Can you work these out from the model? Positions are in its coordinate system, mm. Face numbers are marked on the shaded views. Give positions to 0.01 mm unless a question says otherwise; leave off trailing zeros. Order: outer loops, then holes, each group sorted by start corner. A loop starts at its lowest first (then second) coordinate and runs counter-clockwise, first axis right, second up. Notation, with made-up numbers: M 43.25,13 L 96.25,13 A24 cw 96.25,48 Z; hole C -16,60.25 d6. An arc over 180 degrees is marked long. Answer as a JSON object with one key per item and string values.
```python
from build123d import *

# Parameters (mm, degrees)
SKETCH1_R               = 10
BOSS_EXTRUDE1_DEPTH     = 30
SKETCH2_R               = 2.5
BOSS_EXTRUDE3_DEPTH     = 2
SHELL1_T                = -0.8
SKETCH3_R               = 0.5
CUT_EXTRUDE2_DEPTH      = 34.166247904
CUT_EXTRUDE2_DEPTH_BACK = 34.166247904


with BuildPart() as part:
    # Sketch1 → Boss-Extrude1 (new body)
    with BuildSketch(Plane.XY):
        Circle(SKETCH1_R)
    extrude(amount=BOSS_EXTRUDE1_DEPTH)

    # Sketch2 → Boss-Extrude3 (add)
    with BuildSketch(Plane.XY):
        Circle(SKETCH2_R)
    extrude(amount=-BOSS_EXTRUDE3_DEPTH)

    # Shell1
    shell1_openings = [part.faces().sort_by_distance(p)[0] for p in [
        (0, 0, 30),
        (0, 0, -2),
    ]]
    offset(amount=SHELL1_T, openings=shell1_openings, kind=Kind.INTERSECTION)

    # Sketch3 → Cut-Extrude2 (cut, two sides)
    with BuildSketch(Plane.XY) as cut_extrude2_sk:
        with Locations((5, 0)):
            Circle(SKETCH3_R)
        with Locations((0, -5)):
            Circle(SKETCH3_R)
        with Locations((-5, 0)):
            Circle(SKETCH3_R)
        with Locations((0, 5)):
            Circle(SKETCH3_R)
    extrude(amount=CUT_EXTRUDE2_DEPTH, mode=Mode.SUBTRACT)
    extrude(cut_extrude2_sk.sketch, amount=-CUT_EXTRUDE2_DEPTH_BACK, mode=Mode.SUBTRACT)


solid = part.part
```
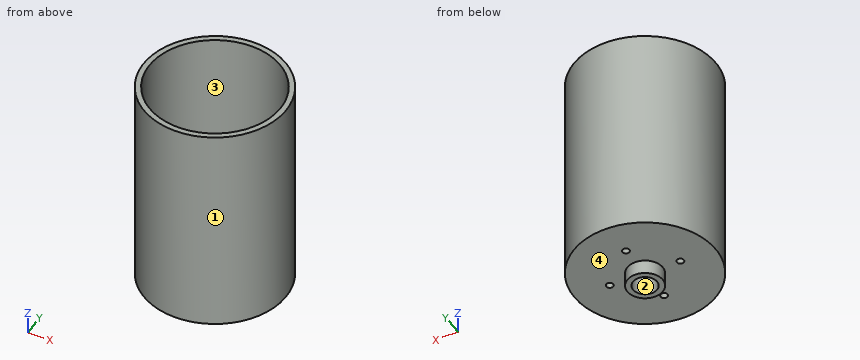
1) I'm going to push flat-ended pins straight in: pin 1 Ø1 at (x, y) = (3.5, 2) entering from +Z; pin 2 Ø10 at (x, z) = (-6.5, 14) entering from +Y; pin 3 Ø8 at (x, z) = (7, 11.5) entering from +Y; pin 4 Ø2 at (x, y) = (0, 0) entering from +Z. Where does each tip first touch, or does it pass through?
Results found:
{"pin 1": "stops at z = 0.8", "pin 2": "stops at y = 9.89", "pin 3": "stops at y = 9.54", "pin 4": "passes through"}
2) I want a section at A-A on y = 0. Write out the boundary of the cut face in (x, z).
Results found:
{"outline": "M -10,0 L -5.5,0 L -5.5,0.8 L -9.2,0.8 L -9.2,30 L -10,30 Z; M -4.5,0 L -2.5,0 L -2.5,-2 L -1.7,-2 L -1.7,0.8 L -4.5,0.8 Z; M 1.7,-2 L 2.5,-2 L 2.5,0 L 4.5,0 L 4.5,0.8 L 1.7,0.8 Z; M 5.5,0 L 10,0 L 10,30 L 9.2,30 L 9.2,0.8 L 5.5,0.8 Z"}
3) I want a section at C-C on z = 17.5. Write out the boundary of the cut face in (x, y).
Results found:
{"outline": "C 0,0 d20; hole C 0,0 d18.4"}
4) I need wall thicknesses on L1, parallel to Y at x = 0, z = 0.6; L2, parallel to Y at x = -0.25, z = 19; L3, parallel to Z at x = -1.75, y = 3.5. Which ranges of each line are inside material? Lowest first, please.
Results found:
{"L1": "y = -10 to -5.5, -4.5 to -1.7, 1.7 to 4.5, 5.5 to 10", "L2": "y = -10 to -9.2, 9.2 to 10", "L3": "z = 0 to 0.8"}
5) Thinking about a two-plate mould opening in X: for the marked faces 1, 2, 3 and 4, which applies, pulls with the +X half, pulls with the -X half, needs draft (parallel to the pull), parting line crosses it, or undercut?
Results found:
{"face 1": "parting line crosses it", "face 2": "undercut", "face 3": "undercut", "face 4": "needs draft"}
6) I want a section at B-B on x = -5. Write out the boundary of the cut face in (y, z), and give its area (3 significant figures).
Results found:
{"outline": "M -8.66,0 L -0.5,0 L -0.5,0.8 L -7.72,0.8 L -7.72,30 L -8.66,30 Z; M 0.5,0 L 8.66,0 L 8.66,30 L 7.72,30 L 7.72,0.8 L 0.5,0.8 Z", "area": "67.8 mm²"}
7) I want a section at D-D on y = 3. Write out the boundary of the cut face in (x, z), and give its area (3 significant figures).
Results found:
{"outline": "M -9.54,0 L 9.54,0 L 9.54,30 L 8.7,30 L 8.7,0.8 L -8.7,0.8 L -8.7,30 L -9.54,30 Z", "area": "64.5 mm²"}
